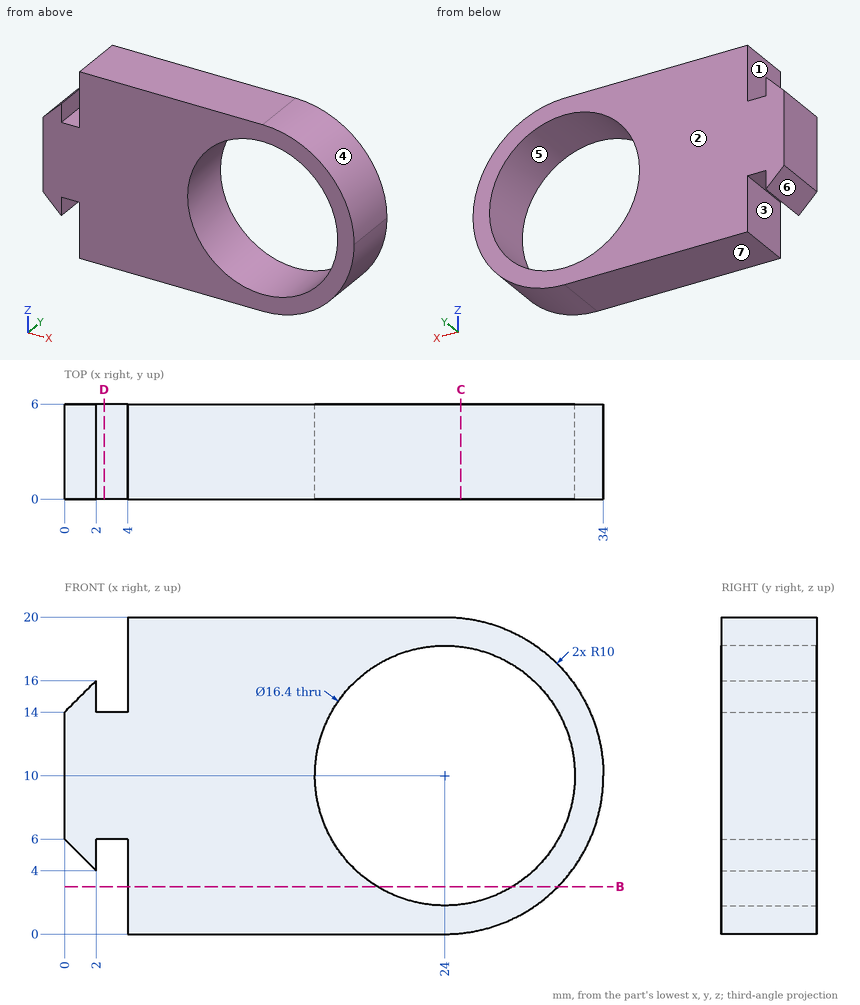
The figure shows three views and two pictorial views of one solid part (mm, origin at its lowest corner). Answer the questions. A direction names the side the tool comes from. Give positions to 0.01 mm unless a question says otherwise; leave off trailing zeros. Loops run counter-clockwise (first coordinate to the right, second up) from the corner with the lowest first, then second, coordinate; pieces in that order, holes last. Notation, with made-up numbers: (-28, 26.5) -> (-22, 26.5) arc R17 ccw to (-22, 49.5) -> close; hole circle Ø11 at (58, 3). An arc over 180 degrees is marked (long way). Put each result on its own line as item: value. Start each with the question number.
Item 1: Find the intervals of material crossed by L1, parallel to X at y = 2.5, z = 10; L2, parallel to X at y = 2.75, z = 15.5; L3, parallel to X at y = 5, z = 11.75, in increasing order. Write a range as [from, to].
Item 2: The mould has two halves that part along X. Classify the marked faces 4, 5, 6 and 7: released by +X, released by -X, zero draft, split by the parting line, or undercut.
Item 3: The part is cut by section D-D (x = 2.5). Give the vertices of the cut face in (y, z), then the cut area to 3 significant figures.
Item 4: Which of the six approach directions +Z, -Z, +X, -X, +Y, -Y give full straight-line access (tool end or side, diameter ignored) to the marked faces 1, 2 and 3?
Item 5: The part is cut by section C-C (x = 25). Give the vertices of the cut face in (y, z), then the cut area to 3 significant figures.
Item 6: The part is cut by section B-B (z = 3). Give the vertices of the cut face in (x, y).
Item 7: Each of these flat-tipped pins is pushed along its axis until it touches: P1, Ø0.6, axis at y = 2.5, z = 15, coming from the +X side; P2, Ø10, axis at x = 24, z = 10, coming from the +Y side; P3, Ø1.8, axis at y = 4.5, z = 3.5, coming from the -X side; P4, Ø1.6, axis at x = 3, y = 3, coming from the -Z side. Where does it stop, or does it pass through?
Answers below:
1. L1: [0, 15.8], [32.2, 34]
1. L2: [1.5, 2], [4, 17.92], [30.08, 32.35]
1. L3: [0, 15.99], [32.01, 33.85]
2. face 4: released by +X
2. face 5: undercut
2. face 6: released by -X
2. face 7: zero draft
3. outline: (0, 6) -> (6, 6) -> (6, 14) -> (0, 14) -> close
3. area: 48.0 mm2
4. face 1: +Z, +Y, -Y
4. face 2: +Z, -Z, +X, -X, +Y
4. face 3: -Z, +Y, -Y
5. outline: (0, 0.05) -> (6, 0.05) -> (6, 1.86) -> (0, 1.86) -> close; (0, 18.14) -> (6, 18.14) -> (6, 19.95) -> (0, 19.95) -> close
5. area: 21.7 mm2
6. outline: (4, 0) -> (19.73, 0) -> (19.73, 6) -> (4, 6) -> close; (28.27, 0) -> (31.14, 0) -> (31.14, 6) -> (28.27, 6) -> close
7. P1: x = 32.83
7. P2: through
7. P3: x = 1.6
7. P4: z = 6
